```python
from build123d import *

# Parameters (mm, degrees)
SKETCH8_W           = 38
SKETCH8_H           = 11
SKETCH8_W_2         = 36.5
SKETCH8_H_2         = 9.5
BOSS_EXTRUDE2_DEPTH = 63
SKETCH9_W           = 38
SKETCH9_H           = 11
BOSS_EXTRUDE3_DEPTH = 1
FILLET1_R           = 1
FILLET2_R           = 1
FILLET3_R           = 1
FILLET4_R           = 1
FILLET5_R           = 1


with BuildPart() as part:
    # Sketch8 → Boss-Extrude2 (new body)
    with BuildSketch(Plane.XY):
        Rectangle(SKETCH8_W, SKETCH8_H)
        Rectangle(SKETCH8_W_2, SKETCH8_H_2, mode=Mode.SUBTRACT)
    extrude(amount=BOSS_EXTRUDE2_DEPTH)

    # Sketch9 → Boss-Extrude3 (add)
    with BuildSketch(Plane.XY.offset(63)):
        Rectangle(SKETCH9_W, SKETCH9_H)
    extrude(amount=BOSS_EXTRUDE3_DEPTH)

    # Fillet1
    fillet1_edges = [part.edges().sort_by_distance(p)[0] for p in [
        (-19, 5.5, 32),
    ]]
    fillet(fillet1_edges, radius=FILLET1_R)

    # Fillet2
    fillet2_edges = [part.edges().sort_by_distance(p)[0] for p in [
        (19, 5.5, 32),
    ]]
    fillet(fillet2_edges, radius=FILLET2_R)

    # Fillet3
    fillet3_edges = [part.edges().sort_by_distance(p)[0] for p in [
        (19, -5.5, 32),
    ]]
    fillet(fillet3_edges, radius=FILLET3_R)

    # Fillet4
    fillet4_edges = [part.edges().sort_by_distance(p)[0] for p in [
        (-19, -5.5, 32),
    ]]
    fillet(fillet4_edges, radius=FILLET4_R)

    # Fillet5
    fillet5_edges = [part.edges().sort_by_distance(p)[0] for p in [
        (-19, 0, 64),
        (-18.707106781, 5.207106781, 64),
        (0, 5.5, 64),
        (18.707106781, 5.207106781, 64),
        (19, 0, 64),
        (18.707106781, -5.207106781, 64),
        (0, -5.5, 64),
        (-18.707106781, -5.207106781, 64),
    ]]
    fillet(fillet5_edges, radius=FILLET5_R)


solid = part.part
```
Read the model definition and answer for the solid it produces. Units are mm, in the model's axes. A direction names the side the tool comes from. Give positions to 0.01 mm unless a question says otherwise; leave off trailing zeros. Order: outer loops, then holes, each group sorted by start corner. A loop starts at its lowest first (then second) coordinate and runs counter-clockwise, first axis right, second up. Notation, with made-up numbers: (86, 87.5) -> (132, 87.5) arc R13 cw to (132, 100.5) -> close; hole circle Ø11 at (49.25, -18). An arc over 180 degrees is marked (long way). One line per item, written item: value. Start each with the question number.
(1) The part is cut by section A-A (z = 17.5). Determine the outline of the cut face in (x, y).
(2) For a pull along X with two mould halves and no side action, classify faces 1 (the flat face through (0, 0, 63)), 2 (the flat face through (19, 0, 31)), 3 (the flat face through (0, -5.5, 31)) as released by +X, released by -X, zero draft, split by the parting line, or undercut.
(3) The part is cut by section B-B (y = 0.5). Determine the outline of the cut face in (x, z).
(4) The part is cut by section C-C (x = 7). Determine the outline of the cut face in (y, z).
(5) A tool of negligible diameter and unlimited length cuts with its end or side. For faces 4 (the flat face through (0, 0, 64)), 5 (the flat face through (18.25, 0, 31)), from which of +Z, -Z, +X, -X, +Y, -Y can it reach the whole face along a straight path? Write none if from no direction.
(6) Straight lines are drawn through the part: L1, parallel to X at y = 1.25, z = 27; L2, parallel to Y at x = 0.5, z = 30; L3, parallel to Z at x = -8, y = -1.5. For each, find the intervals that lie inside material, in ascending order.
Taken from the geometry:
1. outline: (-19, -4.5) arc R1 ccw to (-18, -5.5) -> (18, -5.5) arc R1 ccw to (19, -4.5) -> (19, 4.5) arc R1 ccw to (18, 5.5) -> (-18, 5.5) arc R1 ccw to (-19, 4.5) -> close; hole (-18.25, -4.75) -> (18.25, -4.75) -> (18.25, 4.75) -> (-18.25, 4.75) -> close
2. face 1: undercut
2. face 2: released by +X
2. face 3: zero draft
3. outline: (-19, 0) -> (-18.25, 0) -> (-18.25, 63) -> (18.25, 63) -> (18.25, 0) -> (19, 0) -> (19, 63) arc R1 ccw to (18, 64) -> (-18, 64) arc R1 ccw to (-19, 63) -> close
4. outline: (-5.5, 0) -> (-4.75, 0) -> (-4.75, 63) -> (4.75, 63) -> (4.75, 0) -> (5.5, 0) -> (5.5, 63) arc R1 ccw to (4.5, 64) -> (-4.5, 64) arc R1 ccw to (-5.5, 63) -> close
5. face 4: +Z, +X, -X, +Y, -Y
5. face 5: -Z
6. L1: -19 to -18.25, 18.25 to 19
6. L2: -5.5 to -4.75, 4.75 to 5.5
6. L3: 63 to 64
